Can you work these out from the model? Positions are in its coordinate system, mm. A direction names the side the tool comes from. Round coordinates to 2 decimals unless told otherwise and drop trailing zeros. Loops run counter-clockwise (first coordinate to the right, second up) from the corner with the lowest first, then second, coordinate; pieces in that order, holes last. Notation, with made-up numbers: (51.5, 62) -> (95.5, 62) arc R15 cw to (95.5, 83) -> close; hole circle Ø10 at (-24, 77). An arc over 180 degrees is marked (long way). Write item = value, one per line.
from build123d import *

# Parameters (mm, degrees)
SKETCH_1_W          = 27
SKETCH_1_H          = 18.3
EXTRUDE_1_DEPTH     = 10
SKETCH_2_W          = 22.5
SKETCH_2_H          = 6
CUT_EXTRUDE_1_DEPTH = 10
SKETCH_3_W          = 2
SKETCH_3_H          = 18.3
EXTRUDE_2_DEPTH     = 94


with BuildPart() as part:
    # 草图1 → 凸台-拉伸1 (new body)
    with BuildSketch(Plane(origin=(0, 0, 0), x_dir=(1, 0, 0), z_dir=(0, 1, 0))):
        Rectangle(SKETCH_1_W, SKETCH_1_H)
    extrude(amount=EXTRUDE_1_DEPTH)

    # 草图2 → 切除-拉伸1 (cut)
    with BuildSketch(Plane.XZ):
        with Locations((-0.1, -4.88)):
            Rectangle(SKETCH_2_W, SKETCH_2_H)
        with Locations((-0.1, 4.72)):
            Rectangle(SKETCH_2_W, SKETCH_2_H)
    extrude(amount=-CUT_EXTRUDE_1_DEPTH, mode=Mode.SUBTRACT)

    # 草图3 → 凸台-拉伸2 (add)
    with BuildSketch(Plane.XZ):
        with Locations((-12.5, 0)):
            Rectangle(SKETCH_3_W, SKETCH_3_H)
    extrude(amount=EXTRUDE_2_DEPTH)


solid = part.part
1. Suppose I cut it at B-B, the plane x = -5.5. List the corners of the cut face in (y, z) for me.
Entries:
outline = (0, -9.15) -> (10, -9.15) -> (10, -7.88) -> (0, -7.88) -> close; (0, -1.88) -> (10, -1.88) -> (10, 1.72) -> (0, 1.72) -> close; (0, 7.72) -> (10, 7.72) -> (10, 9.15) -> (0, 9.15) -> close
2. Suppose I cut it at C-C, the plane y = -56.5. List the corners of the cut face in (x, z) for me, and give its area (3 significant figures).
Entries:
outline = (-13.5, -9.15) -> (-11.5, -9.15) -> (-11.5, 9.15) -> (-13.5, 9.15) -> close
area = 36.6 mm²
3. For faces 4 (the flat face through (4, 0, 0)), 5 (the flat face through (-13.5, -41, 0)), 6 (the flat face through (0, 5, 1.72)), which set-ups out of +Z, -Z, +X, -X, +Y, -Y let a thin tool reach every point of the face, with its end or its side?
Entries:
face_4 = +Z, -Z, +X, -Y
face_5 = +Z, -Z, -X, +Y, -Y
face_6 = +Y, -Y
4. I'm going to push a flat-ended pin straight in: pin 1 (3 mm diameter, centred on y = -36.5, z = 3, fed in from +X). Where does the tip first touch, or does it pass through?
Entries:
pin_1 = -11.5
5. Suppose I cut it at A-A, the plane z = 3.25. List the corners of the cut face in (x, y) for me.
Entries:
outline = (-13.5, -94) -> (-11.5, -94) -> (-11.5, 0) -> (-11.35, 0) -> (-11.35, 10) -> (-13.5, 10) -> close; (11.15, 0) -> (13.5, 0) -> (13.5, 10) -> (11.15, 10) -> close
6. We'd pull the mould along X, two halves only. Please class faces 1 (the flat face through (-11.5, -46, 0)), 2 (the flat face through (-12, -15, -9.15)), 3 (the flat face through (0, 5, 7.72)): released by +X, released by -X, zero draft, split by the parting line, or undercut.
Entries:
face_1 = released by +X
face_2 = zero draft
face_3 = undercut
7. I need wall thicknesses on line 1 (X direction, y = 6, z = -2); line 2 (X direction, y = -85.5, z = 1.5); line 3 (Y direction, x = 2.5, z = 8). Which ranges of each line are inside material? Lowest first, please. Write a range as [from, to].
Entries:
line_1 = [-13.5, -11.35], [11.15, 13.5]
line_2 = [-13.5, -11.5]
line_3 = [0, 10]
